Can you work these out from the drawing? Everything is in mm from the part's minimum corner. A direction names the side the tool comes from. Coordinates: 2 decimals unless noted, no trailing zeros. Write each loop counter-clockwise with the first axis right and the second up, starting at its lowest first coordinate (ties: lowest second). Pieces come first, ordered by that corner, then holes. Notation, with made-up numbers: (-3.75, -12.75) -> (34.25, -12.75) arc R21 cw to (34.25, 25.25) -> close; hole circle Ø5 at (51, 88). An arc over 180 degrees is marked (long way). Use a Markdown table: item, result. Add a question column.
Item 1: Will these pins go through, and if not, where does the flat tip stop? pin 1 Ø5 at (x, y) = (21.8, 8.4) entering from +Z; pin 2 Ø5.5 at (x, z) = (32.5, 8) entering from +Y; pin 3 Ø0.6 at (y, z) = (1.5, 1) entering from +X; pin 4 Ø4 at (y, z) = (4.5, 1) entering from +X.
Item 2: On a 3-axis mill with a long thin cutter (end or side, diameter ignored), from which of +Z, -Z, +X, -X, +Y, -Y can I reach the whole of each face in a straight line? I mean the marked faces 4, 5, 6 and 7. Say none if no direction works.
Item 3: Imagine slicing it at C-C, the plane x = 3. Write out the boundary of the cut face in (y, z).
Item 4: If I drill on line 1 along X through (y, z) = (9, 5.55); line 2 along X through (y, z) = (2.5, 1.5); line 3 along Y through (x, z) = (7.5, 9), over which ranges is the centre line in solid material (lowest first)? Write a range as from..to.
Item 5: If we mould it in two halves opening along Z, with no side actions, what happens to the marked faces 1, 2 and 3? For each: pulls with the +Z half, pulls with the -Z half, needs draft (parallel to the pull), parting line crosses it, or undercut.
Item 6: Imagine slicing it at B-B, the plane z = 5.55. Write out the boundary of the cut face in (x, y).
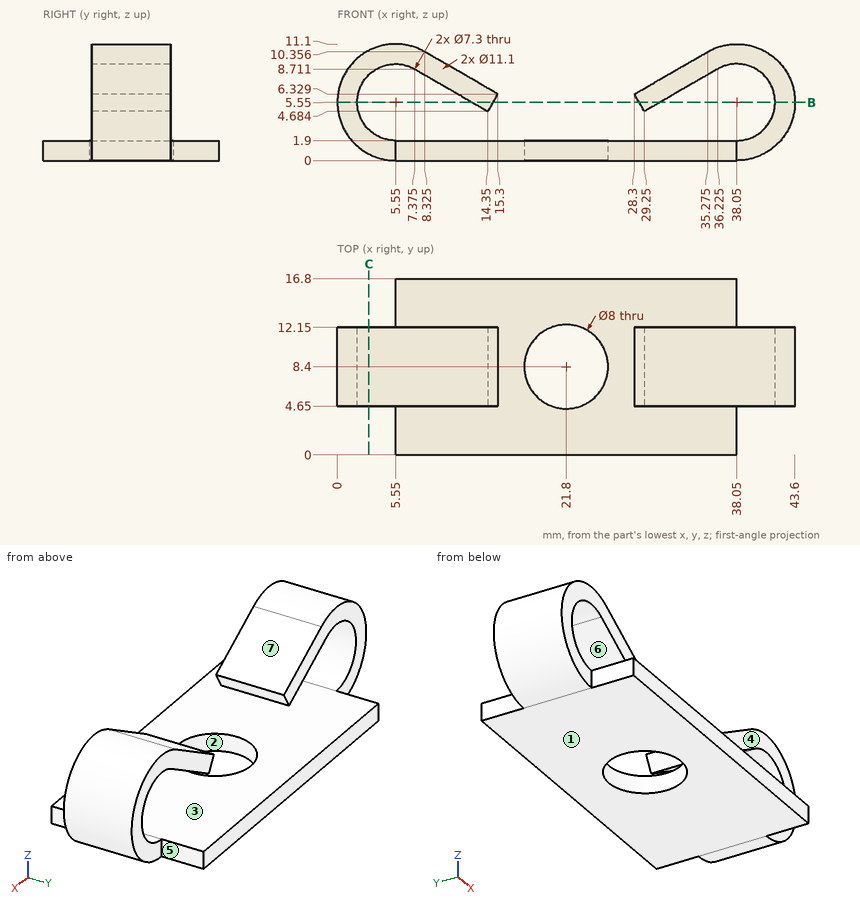
Ans:
| question | item | result |
|---|---|---|
| 1 | pin 1 | passes through |
| 1 | pin 2 | stops at y = 12.15 |
| 1 | pin 3 | stops at x = 38.05 |
| 1 | pin 4 | stops at x = 42.98 |
| 2 | face 4 | +Z, +X, -Y |
| 2 | face 5 | +Z, -Z, +X, +Y |
| 2 | face 6 | +Y, -Y |
| 2 | face 7 | +Z, +Y, -Y |
| 3 | outline | (4.65, 0.62) -> (12.15, 0.62) -> (12.15, 2.94) -> (4.65, 2.94) -> close; (4.65, 8.16) -> (12.15, 8.16) -> (12.15, 10.48) -> (4.65, 10.48) -> close |
| 4 | line 1 | x = 0..1.9, 12.85..14.85, 28.75..30.75, 41.7..43.6 |
| 4 | line 2 | x = 5.55..38.05 |
| 4 | line 3 | y = 4.65..12.15 |
| 5 | face 1 | pulls with the -Z half |
| 5 | face 2 | needs draft |
| 5 | face 3 | undercut |
| 6 | outline | (0, 4.65) -> (1.9, 4.65) -> (1.9, 12.15) -> (0, 12.15) -> close; (12.85, 4.65) -> (14.85, 4.65) -> (14.85, 12.15) -> (12.85, 12.15) -> close; (28.75, 4.65) -> (30.75, 4.65) -> (30.75, 12.15) -> (28.75, 12.15) -> close; (41.7, 4.65) -> (43.6, 4.65) -> (43.6, 12.15) -> (41.7, 12.15) -> close |
